```python
from build123d import *

# Parameters (mm, degrees)
BOSS_EXTRUDE1_DEPTH = 0.6


with BuildPart() as part:
    # Sketch1 → Boss-Extrude1 (new body)
    with BuildSketch(Plane.XY):
        with BuildLine():
            Line((2.7975505, 3.524728529), (2.024608864, 1.107728687))
            ThreePointArc((2.024608864, 1.107728687), (2.015540231, 1.033623325), (2.034280186, 0.961355359))
            ThreePointArc((2.034280186, 0.961355359), (2.249370488, 0.053220369), (2.077469984, -0.864070869))
            ThreePointArc((2.077469984, -0.864070869), (2.074285356, -1.009527687), (2.170509413, -1.118654946))
            Line((2.170509413, -1.118654946), (2.927941172, -1.50902634))
            ThreePointArc((2.927941172, -1.50902634), (3.02857216, -1.63168787), (3.008214578, -1.78903467))
            ThreePointArc((3.008214578, -1.78903467), (2.331985815, -2.609950605), (1.440417044, -3.189858734))
            ThreePointArc((1.440417044, -3.189858734), (1.281779829, -3.192443437), (1.171176469, -3.078692203))
            Line((1.171176469, -3.078692203), (0.868203765, -2.282262523))
            ThreePointArc((0.868203765, -2.282262523), (0.770555129, -2.174408123), (0.625658635, -2.1612615))
            ThreePointArc((0.625658635, -2.1612615), (0, -2.25), (-0.625658635, -2.1612615))
            ThreePointArc((-0.625658635, -2.1612615), (-0.770555129, -2.174408123), (-0.868203765, -2.282262523))
            Line((-0.868203765, -2.282262523), (-1.171176469, -3.078692203))
            ThreePointArc((-1.171176469, -3.078692203), (-1.281779829, -3.192443437), (-1.440417044, -3.189858734))
            ThreePointArc((-1.440417044, -3.189858734), (-2.331985815, -2.609950605), (-3.008214578, -1.78903467))
            ThreePointArc((-3.008214578, -1.78903467), (-3.02857216, -1.63168787), (-2.927941172, -1.50902634))
            Line((-2.927941172, -1.50902634), (-2.170509413, -1.118654946))
            ThreePointArc((-2.170509413, -1.118654946), (-2.074285356, -1.009527687), (-2.077469984, -0.864070869))
            ThreePointArc((-2.077469984, -0.864070869), (-2.249370488, 0.053220369), (-2.034280186, 0.961355359))
            ThreePointArc((-2.034280186, 0.961355359), (-2.015540231, 1.033623325), (-2.024608864, 1.107728687))
            Line((-2.024608864, 1.107728687), (-2.7975505, 3.524728529))
            ThreePointArc((-2.7975505, 3.524728529), (0, -4.5), (2.7975505, 3.524728529))
        make_face()
    extrude(amount=BOSS_EXTRUDE1_DEPTH)


solid = part.part
```
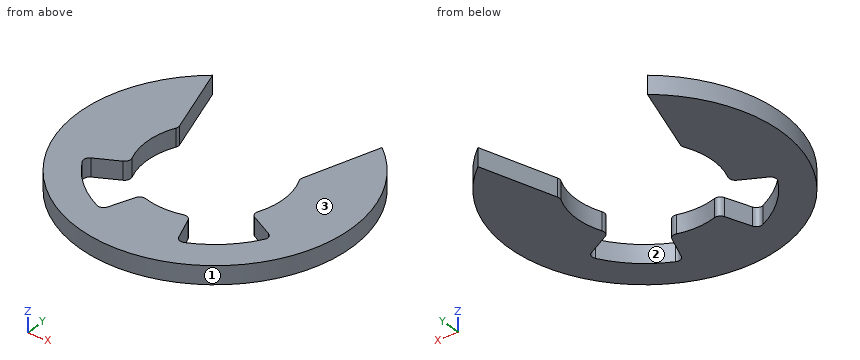
Work out the finished part from the listing and answer in its coordinate system (mm). Face numbers are marked on the shaded views. Round coordinates to 2 decimals unless told otherwise and drop trailing zeros. Write each loop counter-clockwise with the first axis right and the second up, starting at its lowest first coordinate (ties: lowest second). Pieces come first, ordered by that corner, then holes.
1) A cutting plane is placed at C-C on z = 0.1. Determine the outline of the cut face in (x, y), and give its area (3 significant figures).
2) A cutting plane is placed at B-B on x = 0. Determine the outline of the cut face in (y, z), and give its area (3 significant figures).
3) Consider probe 1 along X at (y, z) = (0, 0.25); probe 2 along X at (y, z) = (2.75, 0.35); probe 3 along Y at (x, z) = (-4, 0.35). Determine where each line is inside the solid, lowest interval first.
4) A cutting plane is placed at A-A on y = 0. Determine the outline of the cut face in (x, z).
5) Determine the mould class of the marked faces 1, 2 and 3 for opening direction X: pulls with the +X half, pulls with the -X half, needs draft (parallel to the pull), parting line crosses it, or undercut.
Entries:
1. outline: (-3.01, -1.79) arc R0.2 cw to (-2.93, -1.51) - (-2.17, -1.12) arc R0.2 ccw to (-2.08, -0.86) arc R2.25 cw to (-2.03, 0.96) arc R0.2 ccw to (-2.02, 1.11) - (-2.8, 3.52) arc R4.5 ccw (long way) to (2.8, 3.52) - (2.02, 1.11) arc R0.2 ccw to (2.03, 0.96) arc R2.25 cw to (2.08, -0.86) arc R0.2 ccw to (2.17, -1.12) - (2.93, -1.51) arc R0.2 cw to (3.01, -1.79) arc R3.5 cw to (1.44, -3.19) arc R0.2 cw to (1.17, -3.08) - (0.87, -2.28) arc R0.2 ccw to (0.63, -2.16) arc R2.25 cw to (-0.63, -2.16) arc R0.2 ccw to (-0.87, -2.28) - (-1.17, -3.08) arc R0.2 cw to (-1.44, -3.19) arc R3.5 cw to start
1. area: 30.3 mm2
2. outline: (-4.5, 0) - (-2.25, 0) - (-2.25, 0.6) - (-4.5, 0.6) - close
2. area: 1.35 mm2
3. probe 1: x = -4.5 to -2.25, 2.25 to 4.5
3. probe 2: x = -3.56 to -2.55, 2.55 to 3.56
3. probe 3: y = -2.06 to 2.06
4. outline: (-4.5, 0) - (-2.25, 0) - (-2.25, 0.6) - (-4.5, 0.6) - close; (2.25, 0) - (4.5, 0) - (4.5, 0.6) - (2.25, 0.6) - close
5. face 1: parting line crosses it
5. face 2: undercut
5. face 3: needs draft
